Drawing for the job (mm, zero at the part's lowest x, y, z). A direction names the side the tool comes from. Give positions to 0.01 mm unless a question says otherwise; leave off trailing zeros. Loops run counter-clockwise (first coordinate to the right, second up) from the corner with the lowest first, then second, coordinate; pieces in that order, holes last. Notation, with made-up numbers: M 66,-30 L 89,-30 A29 ccw 89,-7 Z; hole C 21,50.25 d1. An arc over 180 degrees is marked long. Answer in a Markdown table with one row per item. Add a question column.
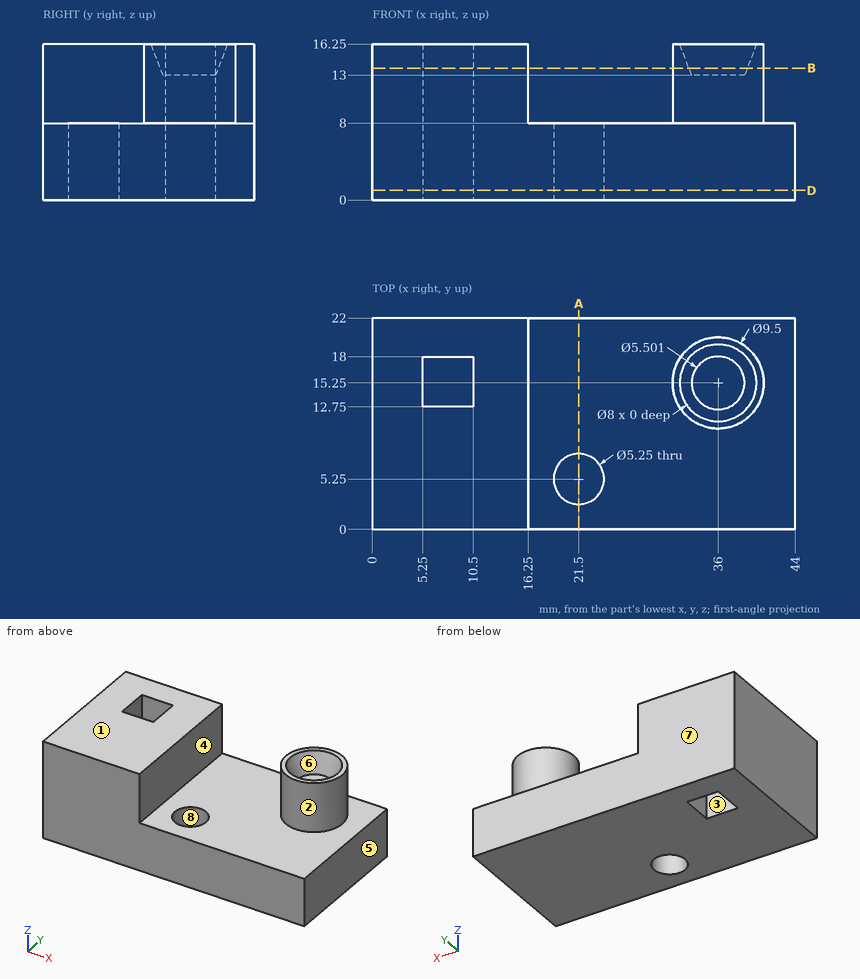
(1) Slice it at B-B, the plane z = 13.75. Give the cut face in (x, y), then the cut area to 3 significant figures.
(2) Slice it at A-A, the plane x = 21.5. Give the cut face in (y, z) (1 decimal), then the cut area to 3 significant figures.
(3) Pull direction X, two halves, no side cores. Call the marked faces 5, 6, 7 and 8: +X half, -X half, draft (parallel to the pull), parting line (faces both ways), or undercut.
(4) Wall check: line 1 (Y direction, x = 21.5, z = 3.5) (1 decimal); line 2 (Y direction, x = 9, z = 5.75); line 3 (X direction, y = 16.5, z = 8.25). Give the ranges that are in metal, low to high.
(5) Slice it at D-D, the plane z = 1. State how many separate pieces and enclosed holes the cut face has, then the cut area to 3 significant figures.
(6) Tool access for the marked faces 1, 2, 3 and 4: list every direction of +Z, -Z, +X, -X, +Y, -Y with a clear straight run to the whole face (end or side of a thin tool).
Solution:
| question | item | result |
|---|---|---|
| 1 | outline | M 0,0 L 16.25,0 L 16.25,22 L 0,22 Z; C 36,15.25 d9.5; hole M 5.25,12.75 L 10.5,12.75 L 10.5,18 L 5.25,18 Z; hole C 36,15.25 d6.08 |
| 1 | area | 372 mm^2 |
| 2 | outline | M 0,0 L 2.6,0 L 2.6,8 L 0,8 Z; M 7.9,0 L 22,0 L 22,8 L 7.9,8 Z |
| 2 | area | 134 mm^2 |
| 3 | face 5 | +X half |
| 3 | face 6 | undercut |
| 3 | face 7 | draft |
| 3 | face 8 | undercut |
| 4 | line 1 | 0 to 2.6, 7.9 to 22 |
| 4 | line 2 | 0 to 12.75, 18 to 22 |
| 4 | line 3 | 0 to 5.25, 10.5 to 16.25, 31.42 to 40.58 |
| 5 | separate pieces | 1 |
| 5 | enclosed holes | 2 |
| 5 | area | 919 mm^2 |
| 6 | face 1 | +Z, +X, -X, +Y, -Y |
| 6 | face 2 | +Z |
| 6 | face 3 | +Z, -Z |
| 6 | face 4 | +Z, +Y, -Y |
